from build123d import *

# Parameters (mm, degrees)
SKETCH1_R           = 1.6
BOSS_EXTRUDE1_DEPTH = 4


with BuildPart() as part:
    # Sketch1 → Boss-Extrude1 (new body)
    with BuildSketch(Plane.XY):
        Polygon((12.5, 35), (-12.5, 35), (-23.334523779, 36.062445841), (-36.062445841, 23.334523779), (-35, 12.5), (-35, -12.5), (-36.062445841, -23.334523779), (-23.334523779, -36.062445841), (-12.5, -35), (12.5, -35), (23.334523779, -36.062445841), (36.062445841, -23.334523779), (35, -12.5), (35, 12.5), (36.062445841, 23.334523779), (23.334523779, 36.062445841), align=None)
        with Locations((22.627416998, 31.112698372)):
            Circle(SKETCH1_R, mode=Mode.SUBTRACT)
        with Locations((31.112698372, 22.627416998)):
            Circle(SKETCH1_R, mode=Mode.SUBTRACT)
        with Locations((22.627416998, -31.112698372)):
            Circle(SKETCH1_R, mode=Mode.SUBTRACT)
        with Locations((31.112698372, -22.627416998)):
            Circle(SKETCH1_R, mode=Mode.SUBTRACT)
        with Locations((-31.112698372, -22.627416998)):
            Circle(SKETCH1_R, mode=Mode.SUBTRACT)
        with Locations((-22.627416998, -31.112698372)):
            Circle(SKETCH1_R, mode=Mode.SUBTRACT)
        with Locations((-22.627416998, 31.112698372)):
            Circle(SKETCH1_R, mode=Mode.SUBTRACT)
        with Locations((-31.112698372, 22.627416998)):
            Circle(SKETCH1_R, mode=Mode.SUBTRACT)
    extrude(amount=BOSS_EXTRUDE1_DEPTH)


solid = part.part
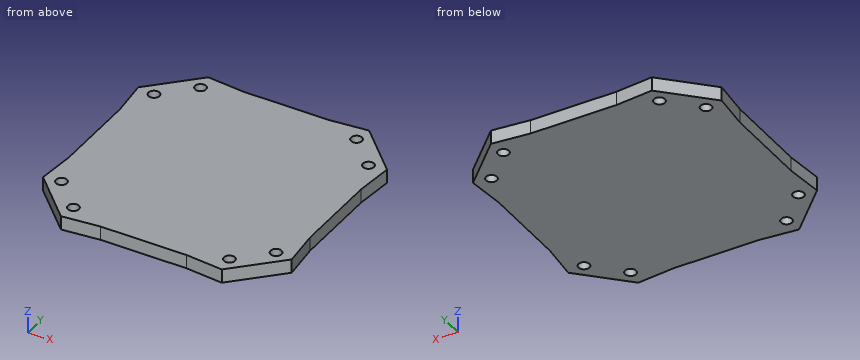
Input: part model. Units: mm. Frame: model coordinates. Coordinates: 2 decimals unless noted, no trailing zeros. Order: outer loops, then holes, each group sorted by start corner. A loop starts at its lowest first (then second) coordinate and runs counter-clockwise, first axis right, second up. Notation, with made-up numbers: M 25,71 L 60,71 A20 ccw 60,92 Z; hole C 48.5,-8 d6. An arc over 180 degrees is marked long. One line per question, with ' | ' between items.
Item 1: Section B-B (x = 4.5). Output: boundary loops of the cut face in (y, z).
Geometry results:
outline: M -35,0 L 35,0 L 35,4 L -35,4 Z
Item 2: Pin query (flat end, axial travel): pin 1 (1.2 mm diameter, centred on y = -0.5, z = 1, fed in from -X); pin 2 (1 mm diameter, centred on y = -18.5, z = 2, fed in from -X); pin 3 (1.2 mm diameter, centred on x = 4.5, z = 2, fed in from -Y). Return the tip coordinate at first contact, or that it passes through.
Geometry results:
pin 1: stops at x = -35 | pin 2: stops at x = -35.64 | pin 3: stops at y = -35
Item 3: Section A-A (z = 2.9). Give the number of separate pieces and of enclosed holes in the cut face, then the cut area to 3 significant figures.
Geometry results:
separate pieces: 1 | enclosed holes: 8 | area: 4,660 mm^2
Item 4: Ray query, line 1 along X through (y, z) = (31, 2.2); line 2 along X through (y, z) = (30, 1.1); line 3 along Y through (x, z) = (32, 3.6). Return the intervals inside material, ascending.
Geometry results:
line 1: x = -28.4 to -24.22, -21.03 to 21.03, 24.22 to 28.4 | line 2: x = -29.4 to -23.78, -21.48 to 21.48, 23.78 to 29.4 | line 3: y = -27.4 to -23.96, -21.3 to 21.3, 23.96 to 27.4
